CAD build for the part. Positions are in the model's coordinates, mm. Face numbers are marked on the shaded views. Give positions to 0.01 mm unless a question says otherwise; leave off trailing zeros. Order: outer loops, then holes, each group sorted by start corner. A loop starts at its lowest first (then second) coordinate and runs counter-clockwise, first axis right, second up. Notation, with made-up numbers: (80, -33) -> (90, -33) arc R19 cw to (90, -16) -> close; hole circle Ø1 at (-26, 60.25). An arc over 180 degrees is marked (long way). Use one line per item in the form item = value. Start each with the question number.
1) Mould opens along Z. For the marked faces 1, 2 and 3 say: pulls with the +Z half, pulls with the -Z half, needs draft (parallel to the pull), parting line crosses it, or undercut.
2) Cut at D-D, the plane y = 4.5. Give the cut face in (x, z).
3) Cut at A-A, the plane z = 6.25. Give the cut face in (x, y).
4) Probe line 1 (Z direction, x = 0, y = -2.2); line 2 (Z direction, x = 0, y = 0.2); line 3 (X direction, y = 1.05, z = 6.25). List the from-to ranges inside material, lowest first.
5) Cut at B-B, the plane y = -2. Give the cut face in (x, z).
6) Cut at C-C, the plane x = 0. Give the cut face in (y, z).
7) Drop flat-ended pins along their axis: P1, Ø3, axis at x = -3.5, y = 4, coming from the -Z side; P2, Ø3, axis at x = 5.5, z = 4, coming from the +Y side; P3, Ø5, axis at x = 0, z = 7.5, coming from the +Y side; P4, Ø4, axis at x = 0, z = 6.25, coming from the +Y side. Give the stop position or say it passes through.
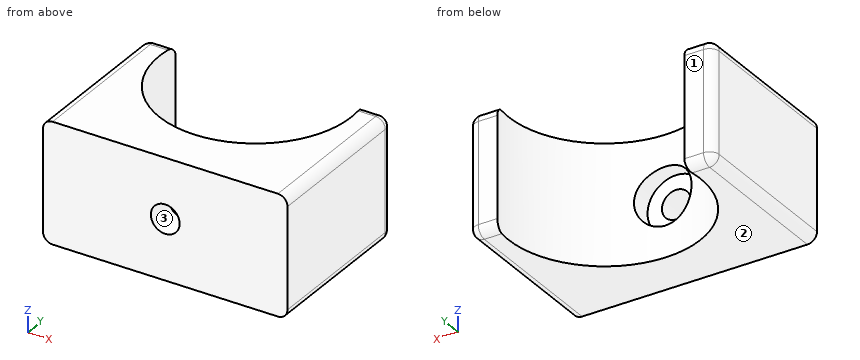
from build123d import *

# Parameters (mm, degrees)
PAD_DEPTH       = 12.5
SKETCH001_R     = 1.5
POCKET_DEPTH    = 17.030262
SKETCH002_R     = 3
POCKET001_DEPTH = 14
FILLET_R        = 1


with BuildPart() as part:
    # Sketch → Pad (new body)
    with BuildSketch(Plane.XY):
        with BuildLine():
            Line((-12.745991, -3.650621), (12.745991, -3.650621))
            Line((12.745991, 13.378641), (12.745991, -3.650621))
            Line((9.745991, 13.378641), (12.745991, 13.378641))
            ThreePointArc((-9.745991, 13.378641), (0, 1.139072), (9.745991, 13.378641))
            Line((-12.745991, 13.378641), (-9.745991, 13.378641))
            Line((-12.745991, -3.650621), (-12.745991, 13.378641))
        make_face()
    extrude(amount=PAD_DEPTH)

    # Sketch001 (on Face1 of Pad) → Pocket (cut, through all)
    with BuildSketch(Plane.XZ.offset(3.650621)):
        with Locations((0, 6.25)):
            Circle(SKETCH001_R)
    extrude(amount=-POCKET_DEPTH, mode=Mode.SUBTRACT)

    # Sketch002 (on Face8 of Pocket) → Pocket001 (cut)
    with BuildSketch(Plane(origin=(0, 13.378641, 0), x_dir=(-1, 0, 0), z_dir=(0, 1, 0))):
        with Locations((0, 6.25)):
            Circle(SKETCH002_R)
    extrude(amount=-POCKET001_DEPTH, mode=Mode.SUBTRACT)

    # Fillet
    fillet_edges = [part.edges().sort_by_distance(p)[0] for p in [
        (12.745991, 4.86401, 12.5),
        (12.745991, 13.378641, 6.25),
        (12.745991, 4.86401, 0),
        (-12.745991, 4.86401, 12.5),
        (-12.745991, 13.378641, 6.25),
        (-12.745991, 4.86401, 0),
        (-11.245991, 13.378641, 12.5),
        (-11.245991, 13.378641, 0),
        (11.245991, 13.378641, 0),
        (11.245991, 13.378641, 12.5),
    ]]
    fillet(fillet_edges, radius=FILLET_R)


solid = part.part
Result:
q1.face_1 = needs draft
q1.face_2 = pulls with the -Z half
q1.face_3 = undercut
q2.outline = (-12.75, 1) arc R1 ccw to (-11.75, 0) -> (-7.48, 0) -> (-7.48, 12.5) -> (-11.75, 12.5) arc R1 ccw to (-12.75, 11.5) -> close; (7.48, 0) -> (11.75, 0) arc R1 ccw to (12.75, 1) -> (12.75, 11.5) arc R1 ccw to (11.75, 12.5) -> (7.48, 12.5) -> close
q3.outline = (-12.75, -3.65) -> (-1.5, -3.65) -> (-1.5, -0.62) -> (-3, -0.62) -> (-3, 1.6) arc R10 cw to (-9.75, 13.38) -> (-11.75, 13.38) arc R1 ccw to (-12.75, 12.38) -> close; (1.5, -3.65) -> (12.75, -3.65) -> (12.75, 12.38) arc R1 ccw to (11.75, 13.38) -> (9.75, 13.38) arc R10 cw to (3, 1.6) -> (3, -0.62) -> (1.5, -0.62) -> close
q4.line_1 = 0 to 4.75, 7.75 to 12.5
q4.line_2 = 0 to 3.25, 9.25 to 12.5
q4.line_3 = -12.75 to -3, 3 to 12.75
q5.outline = (-12.75, 1) arc R1 ccw to (-11.75, 0) -> (11.75, 0) arc R1 ccw to (12.75, 1) -> (12.75, 11.5) arc R1 ccw to (11.75, 12.5) -> (-11.75, 12.5) arc R1 ccw to (-12.75, 11.5) -> close; hole circle Ø3 at (0, 6.25)
q6.outline = (-3.65, 0) -> (1.14, 0) -> (1.14, 3.25) -> (-0.62, 3.25) -> (-0.62, 4.75) -> (-3.65, 4.75) -> close; (-3.65, 7.75) -> (-0.62, 7.75) -> (-0.62, 9.25) -> (1.14, 9.25) -> (1.14, 12.5) -> (-3.65, 12.5) -> close
q7.P1 = through
q7.P2 = 4
q7.P3 = 1.44
q7.P4 = -0.62
